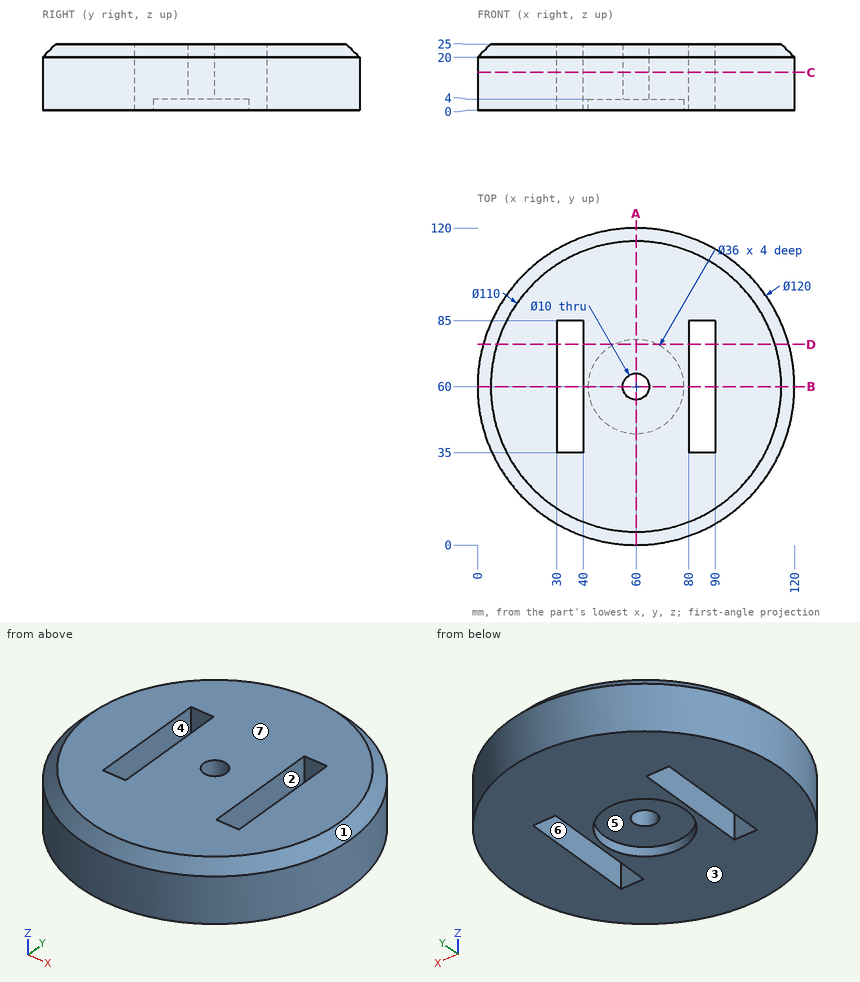
For this review, use the dimensioned drawing (mm, ordinates from the lowest corner) and the shaded views. A direction names the side the tool comes from. Round coordinates to 2 decimals unless told otherwise and drop trailing zeros. Write each loop counter-clockwise with the first axis right and the second up, starting at its lowest first coordinate (ties: lowest second). Pieces come first, ordered by that corner, then holes. Notation, with made-up numbers: (13.5, 62.25) -> (72.5, 62.25) arc R14 ccw to (72.5, 69.25) -> close; hole circle Ø3 at (-29, 39). An arc over 180 degrees is marked (long way). Answer in a Markdown table with one row per item.
Q1. Take a section at B-B, the plane y = 60. State the section outline as (x, z) points.
The answers:
| item | result |
|---|---|
| outline | (0, 0) -> (30, 0) -> (30, 25) -> (5, 25) -> (0, 20) -> close; (40, 0) -> (42, 0) -> (42, 4) -> (55, 4) -> (55, 25) -> (40, 25) -> close; (65, 4) -> (78, 4) -> (78, 0) -> (80, 0) -> (80, 25) -> (65, 25) -> close; (90, 0) -> (120, 0) -> (120, 20) -> (115, 25) -> (90, 25) -> close |
Q2. For the marked faces 5, 6 and 7, list the 3-axis set-ups (+Z, -Z, +X, -X, +Y, -Y) from which the entire face can be reached by the end or side of a thin tool; tool diameter is ignored.
The answers:
| item | result |
|---|---|
| face 5 | -Z |
| face 6 | +Z, -Z |
| face 7 | +Z, +X, -X, +Y, -Y |
Q3. Take a section at C-C, the plane z = 14.25. State the section outline as (x, y) points, then the cut area to 3 significant figures.
The answers:
| item | result |
|---|---|
| outline | circle Ø120 at (60, 60); hole (30, 35) -> (40, 35) -> (40, 85) -> (30, 85) -> close; hole circle Ø10 at (60, 60); hole (80, 35) -> (90, 35) -> (90, 85) -> (80, 85) -> close |
| area | 10,200 mm² |
Q4. To check wall thickness, follow L1, parallel to Y at x = 60, z = 16.25; L2, parallel to X at y = 73.5, z = 5.5; L3, parallel to X at y = 83, z = 19. State the ranges of each line that lie inside material, in increasing order. Write a range as [from, to].
The answers:
| item | result |
|---|---|
| L1 | [0, 55], [65, 120] |
| L2 | [1.54, 30], [40, 80], [90, 118.46] |
| L3 | [4.58, 30], [40, 80], [90, 115.42] |
Q5. Draft analysis for pull direction X (two halves, no side actions). For the marked faces 1, 2, 3 and 4, state which applies: +X half, -X half, draft (parallel to the pull), parting line (faces both ways), or undercut.
The answers:
| item | result |
|---|---|
| face 1 | parting line |
| face 2 | undercut |
| face 3 | draft |
| face 4 | undercut |
Q6. Take a section at D-D, the plane y = 76. Count the separate pieces of the cut face and the enclosed holes in it, then the cut area to 3 significant figures.
The answers:
| item | result |
|---|---|
| separate pieces | 3 |
| enclosed holes | 0 |
| area | 2,300 mm² |
Q7. Take a section at A-A, the plane x = 60. State the section outline as (y, z) points.
The answers:
| item | result |
|---|---|
| outline | (0, 0) -> (42, 0) -> (42, 4) -> (55, 4) -> (55, 25) -> (5, 25) -> (0, 20) -> close; (65, 4) -> (78, 4) -> (78, 0) -> (120, 0) -> (120, 20) -> (115, 25) -> (65, 25) -> close |
Q8. Clearance check with flat-ended pins moving along their axes: pin 1 Ø1.5 at (y, z) = (34, 14) entering from +X; pin 2 Ø7.5 at (y, z) = (52.5, 8.5) entering from +X; pin 3 Ø18 at (x, y) = (55.5, 64.5) entering from -Z; pin 4 Ø9 at (x, y) = (60, 60) entering from -Z. State where each tip first meets the part, or that it passes through.
The answers:
| item | result |
|---|---|
| pin 1 | x = 114.43 |
| pin 2 | x = 119.88 |
| pin 3 | z = 4 |
| pin 4 | through |
